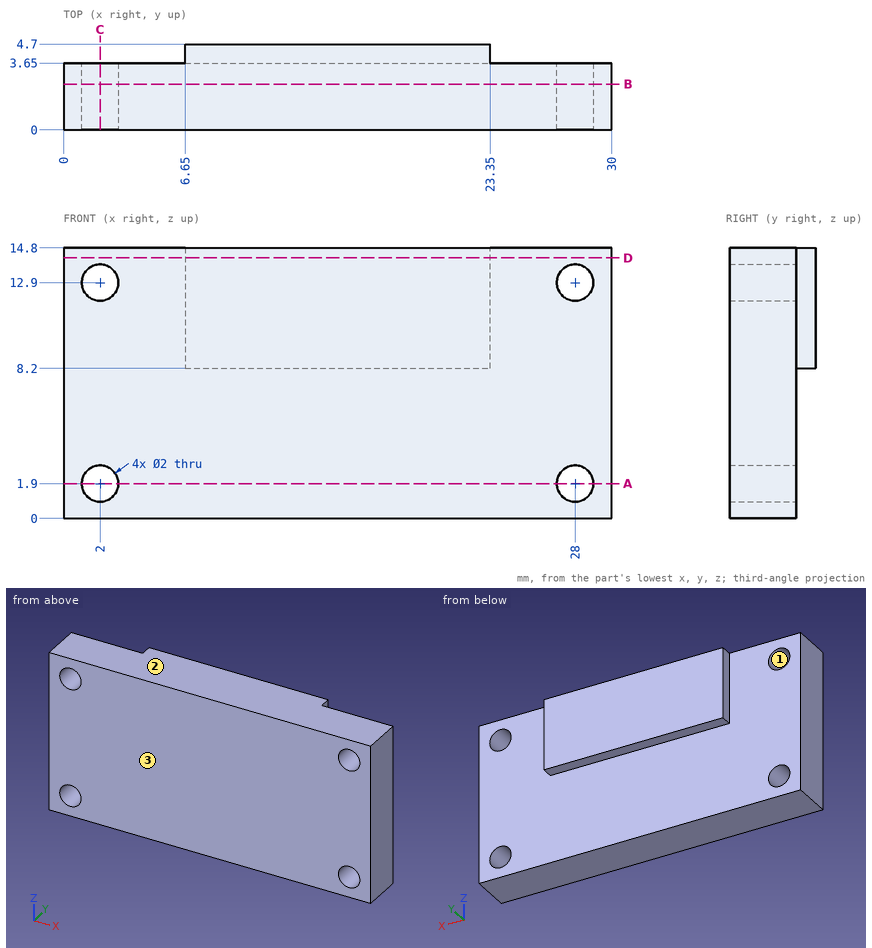
Answer from the drawing. Dimensions are ordinates in mm from the lowest x, y and z of the part. Give positions to 0.01 mm unless a question says otherwise; leave off trailing zeros. Order: outer loops, then holes, each group sorted by start corner. A loop starts at its lowest first (then second) coordinate and runs counter-clockwise, first axis right, second up. Notation, with made-up numbers: (-27.75, 53.5) -> (-8.75, 53.5) arc R24 ccw to (-8.75, 73.5) -> close; hole circle Ø5 at (56.5, -24.75). An arc over 180 degrees is marked (long way). One line per item, written item: value. Start each with the question number.
(1) The part is cut by section D-D (z = 14.25). Determine the outline of the cut face in (x, y), and give its area (3 significant figures).
(2) The part is cut by section B-B (y = 2.5). Determine the outline of the cut face in (x, z).
(3) Straight lines are drawn through the part: L1, parallel to X at y = 1.25, z = 12.9; L2, parallel to Z at x = 28, y = 2; L3, parallel to X at y = 1.4, z = 2.75. For each, find the intervals that lie inside material, in ascending order.
(4) Flat-ended cylindrical pins translate along their axes: P1, Ø1.8, axis at x = 28, z = 1.9, coming from the +Y side; P2, Ø1.2, axis at x = 14.5, y = 4.5, coming from the -Z side; P3, Ø2, axis at x = 25, z = 13, coming from the +Y side. Find the tip coordinate at first contact, or state that the pin passes through.
(5) For a pull along Z with two mould halves and no side action, classify the marked faces 1, 2 and 3 as released by +Z, released by -Z, zero draft, split by the parting line, or undercut.
(6) The part is cut by section A-A (z = 1.9). Determine the outline of the cut face in (x, y).
(7) The part is cut by section C-C (x = 2). Determine the outline of the cut face in (y, z).
Taken from the geometry:
1. outline: (0, 0) -> (30, 0) -> (30, 3.65) -> (23.35, 3.65) -> (23.35, 4.7) -> (6.65, 4.7) -> (6.65, 3.65) -> (0, 3.65) -> close
1. area: 127 mm^2
2. outline: (0, 0) -> (30, 0) -> (30, 14.8) -> (0, 14.8) -> close; hole circle Ø2 at (2, 1.9); hole circle Ø2 at (2, 12.9); hole circle Ø2 at (28, 1.9); hole circle Ø2 at (28, 12.9)
3. L1: 0 to 1, 3 to 27, 29 to 30
3. L2: 0 to 0.9, 2.9 to 11.9, 13.9 to 14.8
3. L3: 0 to 1.47, 2.53 to 27.47, 28.53 to 30
4. P1: through
4. P2: z = 8.2
4. P3: y = 3.65
5. face 1: undercut
5. face 2: released by +Z
5. face 3: zero draft
6. outline: (0, 0) -> (1, 0) -> (1, 3.65) -> (0, 3.65) -> close; (3, 0) -> (27, 0) -> (27, 3.65) -> (3, 3.65) -> close; (29, 0) -> (30, 0) -> (30, 3.65) -> (29, 3.65) -> close
7. outline: (0, 0) -> (3.65, 0) -> (3.65, 0.9) -> (0, 0.9) -> close; (0, 2.9) -> (3.65, 2.9) -> (3.65, 11.9) -> (0, 11.9) -> close; (0, 13.9) -> (3.65, 13.9) -> (3.65, 14.8) -> (0, 14.8) -> close
